```python
from build123d import *

# Parameters (mm, degrees)
F1_DEPTH = 5.0038
F2_R     = 3.175
F3_R     = 8.001
F4_DEPTH = 5.0038
F5_W     = 1.016
F5_H     = 5.0038
F6_DEPTH = 5.0038
F7_R     = 2.3876
F8_DEPTH = 5.0038


with BuildPart() as f1:
    # F0 (on Front) → F1 (new body)
    with BuildSketch(Plane.XZ):
        with BuildLine():
            ThreePointArc((9.9949, 48.006), (-5.4790676118, 56.3652968673), (-3.9878, 38.841095354))
            ThreePointArc((-3.9878, 38.841095354), (-0.5154258333, 38.0243988148), (3.0226, 38.4790951905))
            ThreePointArc((3.0226, 38.4790951905), (8.0656249215, 42.1031430108), (9.9949, 48.006))
        make_face()
        with BuildLine():
            Line((-3.9878, 38.841095354), (-3.9878, 9.164904646))
            ThreePointArc((-3.9878, 9.164904646), (-8.9961822265, -4.3550810966), (4.7152403545, -8.8127484027))
            Line((4.7152403545, -8.8127484027), (16.0724023653, -2.7361255174))
            ThreePointArc((16.0724023653, -2.7361255174), (18.5431093303, 6.4043007502), (9.270553305, 8.3204140086))
            ThreePointArc((9.270553305, 8.3204140086), (5.1603136206, 8.0483265237), (3.0226, 11.5694459962))
            Line((3.0226, 11.5694459962), (3.0226, 38.4790951905))
            ThreePointArc((3.0226, 38.4790951905), (-0.5154258333, 38.0243988148), (-3.9878, 38.841095354))
        make_face()
    extrude(amount=F1_DEPTH)

    # F2
    f2_edges = [f1.edges().sort_by_distance(p)[0] for p in [
        (-3.9878, -2.5019, 38.841095),
        (3.0226, -2.5019, 38.479095),
        (-3.9878, -2.5019, 9.164905),
    ]]
    fillet(f2_edges, radius=F2_R)

    # F3 (on face) → F4 (cut)
    with BuildSketch(Plane.XZ.offset(5.0038)):
        with Locations((0, 48.006)):
            Circle(F3_R)
        Circle(F3_R)
    extrude(amount=-F4_DEPTH, mode=Mode.SUBTRACT)

    # F5 (on face) → F6 (cut)
    with BuildSketch(Plane.XZ.offset(5.0038)):
        with Locations((2.5146, 31.0007)):
            Rectangle(F5_W, F5_H)
    extrude(amount=-F6_DEPTH, mode=Mode.SUBTRACT)

    # F7 (on face) → F8 (cut)
    with BuildSketch(Plane.XZ.offset(5.0038)):
        with Locations((13.0048, 2.9972)):
            Circle(F7_R)
    extrude(amount=-F8_DEPTH, mode=Mode.SUBTRACT)


solid = f1.part
```
Design review of the part built by this model. Coordinates are the model's own, in mm. A direction names the side the tool comes from. Round coordinates to 2 decimals unless told otherwise and drop trailing zeros. Write each loop counter-clockwise with the first axis right and the second up, starting at its lowest first coordinate (ties: lowest second). Pieces come first, ordered by that corner, then holes.
Item 1: For faces 1 (the flat face through (2.5, -5.004, 19.1)), 2 (the cylindrical face through (-4.384, -2.537, 38.49)), 3 (the flat face through (2.5, 0, 19.1)), 4 (the flat face through (3.023, -2, 20)), 5 (the cylindrical face through (5.214, -2.467, 8.021)), list the 3-axis set-ups (+Z, -Z, +X, -X, +Y, -Y) from which the entire face can be reached by the end or side of a thin tool; tool diameter is ignored.
Item 2: We need section C-C on y = -1.7. State how many separate pieces and enclosed holes the cut face has, and give its area (3 significant figures).
Item 3: For probe 1 along Z at (x, y) = (0, -1.9) (3 decimals); probe 2 along Z at (x, y) = (-3.25, -4.1); probe 3 along X at (y, z) = (-2.2, 18.5), list the stretches that pass through material, from the lowest coordinate up.
Item 4: We need section B-B on x = 0. Write out the cut boundary in (y, z) (3 decimals).
Item 5: Clearance check with flat-ended pins moving along their axes: pin 1 Ø3 at (y, z) = (-2.5, 35) entering from +X; pin 2 Ø1.5 at (x, y) = (2, -4) entering from -Z; pin 3 Ø0.5 at (x, y) = (2.5, -3.5) entering from +Z; pin 4 Ø14.5 at (x, z) = (0, 48.006) entering from -Y. State where each tip first meets the part, or that it passes through.
Item 6: We need section A-A on z = 0. Write out the cut boundary in (x, y), and give its area (3 significant figures).
Item 7: We need section D-D on x = 6.5. Write out the cut boundary in (y, z).
Returned:
1. face 1: +Z, -Z, +X, -X, -Y
1. face 2: -X, +Y, -Y
1. face 3: +Z, -Z, +X, -X, +Y
1. face 4: +X, +Y, -Y
1. face 5: +Y, -Y
2. separate pieces: 1
2. enclosed holes: 3
2. area: 529 mm2
3. probe 1: z = -9.995 to -8.001, 8.001 to 40.005, 56.007 to 58.001
3. probe 2: z = -9.45 to -7.31, 7.31 to 40.69, 55.32 to 57.46
3. probe 3: x = -3.99 to 3.02
4. outline: (-5.004, -9.995) - (0, -9.995) - (0, -8.001) - (-5.004, -8.001) - close; (-5.004, 8.001) - (0, 8.001) - (0, 40.005) - (-5.004, 40.005) - close; (-5.004, 56.007) - (0, 56.007) - (0, 58.001) - (-5.004, 58.001) - close
5. pin 1: stops at x = 3.02
5. pin 2: stops at z = -9.92
5. pin 3: stops at z = 57.74
5. pin 4: passes through
6. outline: (-9.99, -5) - (-8, -5) - (-8, 0) - (-9.99, 0) - close; (8, -5) - (18.78, -5) - (18.78, 0) - (8, 0) - close
6. area: 63.9 mm2
7. outline: (-5, -7.86) - (0, -7.86) - (0, -4.67) - (-5, -4.67) - close; (-5, 4.67) - (0, 4.67) - (0, 7.63) - (-5, 7.63) - close; (-5, 40.41) - (0, 40.41) - (0, 43.34) - (-5, 43.34) - close; (-5, 52.67) - (0, 52.67) - (0, 55.6) - (-5, 55.6) - close
